Work out the finished part from the listing and answer in its coordinate system (mm). A direction names the side the tool comes from. Coordinates: 2 decimals unless noted, no trailing zeros. Write each loop counter-clockwise with the first axis right and the second up, starting at its lowest first coordinate (ties: lowest second). Pieces come first, ordered by that corner, then holes. Notation, with made-up numbers: (55.25, -35.75) - (107.25, -35.75) arc R17 ccw to (107.25, -30.75) - close; hole circle Ø3 at (37, 9). An arc over 180 degrees is marked (long way). Use one line per item in the form item = value. Start each with the question number.
Item 1: A cutting plane is placed at D-D (z = -10). Give the number of separate pieces and of enclosed holes in the cut face, then the cut area to 3 significant figures.
Item 2: For faces 1 (the flat face through (16.303, -1, -10)), 2 (the flat face through (37.803, 27, -10)), 3 (the flat face through (4, -1, -12.75)), 4 (the flat face through (4, -1, -7.25)), 5 (the flat face through (43.303, 18, -10)), determine the directions among +Z, -Z, +X, -X, +Y, -Y from which every point of the face is accessible in a straight line to the end or side of a thin tool.
Item 3: Consider probe 1 along X at (y, z) = (25, -10); probe 2 along X at (y, z) = (3.25, -10); probe 3 along X at (y, z) = (27, -1.5). Determine where each line is inside the solid, lowest interval first.
Item 4: A cutting plane is placed at C-C (y = 12). Write down the section's boundary in (x, z), then the cut area to 3 significant figures.
Item 5: A cutting plane is placed at B-B (z = -2.5). Write down the section's boundary in (x, y).
Item 6: A cutting plane is placed at A-A (y = 25.5). Write down the section's boundary in (x, z), then the cut area to 3 significant figures.
Item 7: Determine the mould class of faces 6 (the flat face through (36, 29, -12)), 7 (the flat face through (39, -1, -7.25)), 8 (the flat face through (40, -2.5, -10)) for opening direction Y: released by +Y, released by -Y, zero draft, split by the parting line, or undercut.
Item 8: Given pin 1 (0.8 mm diameter, centred on x = 4, y = -1, fed in from -Z); pin 2 (0.8 mm diameter, centred on x = 11.5, y = -1.5, fed in from +Z); pin 3 (4.5 mm diameter, centred on x = 8.8, z = -10, fed in from -Y), each flat-ended and moving along its own axis, determine where each tip first touches the part or whether it passes through.
from build123d import *

# Parameters (mm, degrees)
SKETCH1_W           = 44
SKETCH1_H           = 20
BOSS_EXTRUDE1_DEPTH = 39
SKETCH3_W           = 44
SKETCH3_H           = 5.5
BOSS_EXTRUDE5_DEPTH = 2.5
SKETCH2_R           = 2.8
CUT_EXTRUDE1_DEPTH  = 42.5
SKETCH4_R           = 5
CUT_EXTRUDE2_DEPTH  = 34
SKETCH5_W           = 8
SKETCH5_H           = 4.5
CUT_EXTRUDE3_DEPTH  = 21
SKETCH6_W           = 10
SKETCH6_H           = 5.5
CUT_EXTRUDE4_DEPTH  = 2.5


with BuildPart() as part:
    # Sketch1 → Boss-Extrude1 (new body)
    with BuildSketch(Plane(origin=(0, 0, 0), x_dir=(1, 0, 0), z_dir=(0, 1, 0))):
        with Locations((21.30324178, 10)):
            Rectangle(SKETCH1_W, SKETCH1_H)
    extrude(amount=BOSS_EXTRUDE1_DEPTH)

    # Sketch3 → Boss-Extrude5 (add)
    with BuildSketch(Plane.XZ):
        with Locations((21.30324178, -10)):
            Rectangle(SKETCH3_W, SKETCH3_H)
    extrude(amount=BOSS_EXTRUDE5_DEPTH)

    # Sketch2 → Cut-Extrude1 (cut, through all)
    with BuildSketch(Plane(origin=(0, 39, 0), x_dir=(1, 0, 0), z_dir=(0, 1, 0))):
        with Locations((8.80324178, 10)):
            Circle(SKETCH2_R)
        with Locations((33.80324178, 10)):
            Circle(SKETCH2_R)
        with Locations((21.30324178, 10)):
            Circle(SKETCH2_R)
    extrude(amount=-CUT_EXTRUDE1_DEPTH, mode=Mode.SUBTRACT)

    # Sketch4 → Cut-Extrude2 (cut)
    with BuildSketch(Plane(origin=(0, 39, 0), x_dir=(1, 0, 0), z_dir=(0, 1, 0))):
        with Locations((21.30324178, 10)):
            Circle(SKETCH4_R)
    extrude(amount=-CUT_EXTRUDE2_DEPTH, mode=Mode.SUBTRACT)

    # Sketch5 → Cut-Extrude3 (cut, through all)
    with BuildSketch(Plane(origin=(0, 0, -20), x_dir=(-1, 0, 0), z_dir=(0, 0, -1))):
        with Locations((-33.80324178, 26.75)):
            Rectangle(SKETCH5_W, SKETCH5_H)
        with Locations((-8.80324178, 26.75)):
            Rectangle(SKETCH5_W, SKETCH5_H)
    extrude(amount=-CUT_EXTRUDE3_DEPTH, mode=Mode.SUBTRACT)

    # Sketch6 → Cut-Extrude4 (cut)
    with BuildSketch(Plane.XZ.offset(2.5)):
        with Locations((21.30324178, -10)):
            Rectangle(SKETCH6_W, SKETCH6_H)
    extrude(amount=-CUT_EXTRUDE4_DEPTH, mode=Mode.SUBTRACT)


solid = part.part
Answer:
q1.separate_pieces = 4
q1.enclosed_holes = 0
q1.area = 947 mm²
q2.face_1 = +Z, -Z, -Y
q2.face_2 = +Z, -Z
q2.face_3 = -Z, +X, -X, -Y
q2.face_4 = +Z, +X, -X, -Y
q2.face_5 = +Z, -Z, +X, +Y, -Y
q3.probe_1 = -0.7 to 4.8, 12.8 to 16.3, 26.3 to 29.8, 37.8 to 43.3
q3.probe_2 = -0.7 to 6, 11.6 to 18.5, 24.1 to 31, 36.6 to 43.3
q3.probe_3 = -0.7 to 4.8, 12.8 to 29.8, 37.8 to 43.3
q4.outline = (-0.7, -20) - (43.3, -20) - (43.3, 0) - (-0.7, 0) - close; hole circle Ø5.6 at (8.8, -10); hole circle Ø10 at (21.3, -10); hole circle Ø5.6 at (33.8, -10)
q4.area = 752 mm²
q5.outline = (-0.7, 0) - (43.3, 0) - (43.3, 39) - (-0.7, 39) - close; hole (4.8, 24.5) - (12.8, 24.5) - (12.8, 29) - (4.8, 29) - close; hole (29.8, 24.5) - (37.8, 24.5) - (37.8, 29) - (29.8, 29) - close
q6.outline = (-0.7, -20) - (4.8, -20) - (4.8, 0) - (-0.7, 0) - close; (12.8, -20) - (29.8, -20) - (29.8, 0) - (12.8, 0) - close; (37.8, -20) - (43.3, -20) - (43.3, 0) - (37.8, 0) - close; hole circle Ø10 at (21.3, -10)
q6.area = 481 mm²
q7.face_6 = undercut
q7.face_7 = zero draft
q7.face_8 = released by -Y
q8.pin_1 = -12.75
q8.pin_2 = -7.25
q8.pin_3 = through
